```python
from build123d import *

# Parameters (mm, degrees)
SKETCH_1_R      = 2.5
EXTRUDE_1_DEPTH = 3


with BuildPart() as part:
    # 草图1 → 凸台-拉伸1 (new body)
    with BuildSketch(Plane(origin=(0, 0, 0), x_dir=(0, 0, -1), z_dir=(1, 0, 0))):
        with BuildLine():
            Line((0, -10), (175, -10))
            Line((175, -10), (200, -10))
            ThreePointArc((200, -10), (203.535533906, -8.535533906), (205, -5))
            Line((205, -5), (205, 45))
            ThreePointArc((205, 45), (204.472135955, 47.236067977), (203, 49))
            Line((203, 49), (177.666666667, 68))
            ThreePointArc((177.666666667, 68), (174.828944327, 69.486832981), (171.666666667, 70))
            Line((171.666666667, 70), (95, 70))
            ThreePointArc((95, 70), (91.207635036, 69.252997784), (87.98185108, 67.123593597))
            Line((87.98185108, 67.123593597), (32.919623175, 12.876406403))
            ThreePointArc((32.919623175, 12.876406403), (29.693839218, 10.747002216), (25.901474255, 10))
            Line((25.901474255, 10), (0, 10))
            ThreePointArc((0, 10), (-10, 0), (0, -10))
        make_face()
        Circle(SKETCH_1_R, mode=Mode.SUBTRACT)
        with Locations((95, 0)):
            Circle(SKETCH_1_R, mode=Mode.SUBTRACT)
        with Locations((95, 60)):
            Circle(SKETCH_1_R, mode=Mode.SUBTRACT)
        with Locations((200, 45)):
            Circle(SKETCH_1_R, mode=Mode.SUBTRACT)
        with Locations((200, -5)):
            Circle(SKETCH_1_R, mode=Mode.SUBTRACT)
        with Locations((185, 45)):
            Circle(SKETCH_1_R, mode=Mode.SUBTRACT)
        with Locations((185, -5)):
            Circle(SKETCH_1_R, mode=Mode.SUBTRACT)
        with BuildLine():
            Line((46.298034327, 0), (75.635083269, 0))
            ThreePointArc((75.635083269, 0), (78.696945447, 1.047152925), (80.476312452, 3.75))
            ThreePointArc((80.476312452, 3.75), (84.393398282, 10.606601718), (91.25, 14.523687548))
            ThreePointArc((91.25, 14.523687548), (93.952847075, 16.303054553), (95, 19.364916731))
            Line((95, 19.364916731), (95, 40.635083269))
            ThreePointArc((95, 40.635083269), (93.952847075, 43.696945447), (91.25, 45.476312452))
            ThreePointArc((91.25, 45.476312452), (89.208124255, 46.163303308), (87.285721083, 47.135712192))
            ThreePointArc((87.285721083, 47.135712192), (84.121274015, 47.812324342), (81.205220318, 46.409413055))
            Line((81.205220318, 46.409413055), (42.788959867, 8.561796798))
            ThreePointArc((42.788959867, 8.561796798), (41.671535435, 3.103817518), (46.298034327, 0))
        make_face(mode=Mode.SUBTRACT)
        with BuildLine():
            Line((108.2, 43.85), (121.333333333, 34))
            ThreePointArc((121.333333333, 34), (123.333333333, 30), (121.333333333, 26))
            Line((121.333333333, 26), (108.2, 16.15))
            ThreePointArc((108.2, 16.15), (106.105572809, 15.961145618), (105, 17.75))
            Line((105, 17.75), (105, 42.25))
            ThreePointArc((105, 42.25), (106.105572809, 44.038854382), (108.2, 43.85))
        make_face(mode=Mode.SUBTRACT)
        with BuildLine():
            Line((122.666666667, 50), (147.333333333, 50))
            ThreePointArc((147.333333333, 50), (149.230699929, 48.632455532), (148.533333333, 46.4))
            Line((148.533333333, 46.4), (138, 38.5))
            ThreePointArc((138, 38.5), (135, 37.5), (132, 38.5))
            Line((132, 38.5), (121.466666667, 46.4))
            ThreePointArc((121.466666667, 46.4), (120.769300071, 48.632455532), (122.666666667, 50))
        make_face(mode=Mode.SUBTRACT)
        with BuildLine():
            Line((163.201700099, 40.901275074), (163.201700099, 19.098724926))
            ThreePointArc((163.201700099, 19.098724926), (162.09612729, 17.309870544), (160.001700099, 17.498724926))
            Line((160.001700099, 17.498724926), (148.666666667, 26))
            ThreePointArc((148.666666667, 26), (146.666666667, 30), (148.666666667, 34))
            Line((148.666666667, 34), (160.001700099, 42.501275074))
            ThreePointArc((160.001700099, 42.501275074), (162.09612729, 42.690129456), (163.201700099, 40.901275074))
        make_face(mode=Mode.SUBTRACT)
        with BuildLine():
            Line((121.466666667, 13.6), (132, 21.5))
            ThreePointArc((132, 21.5), (135, 22.5), (138, 21.5))
            Line((138, 21.5), (148.533333333, 13.6))
            ThreePointArc((148.533333333, 13.6), (149.230699929, 11.367544468), (147.333333333, 10))
            Line((147.333333333, 10), (122.666666667, 10))
            ThreePointArc((122.666666667, 10), (120.769300071, 11.367544468), (121.466666667, 13.6))
        make_face(mode=Mode.SUBTRACT)
        with BuildLine():
            Line((115, 63), (165, 63))
            ThreePointArc((165, 63), (168, 60), (165, 57))
            Line((165, 57), (115, 57))
            ThreePointArc((115, 57), (112, 60), (115, 63))
        make_face(mode=Mode.SUBTRACT)
        with BuildLine():
            Line((115, 3), (165, 3))
            ThreePointArc((165, 3), (168, 0), (165, -3))
            Line((165, -3), (115, -3))
            ThreePointArc((115, -3), (112, 0), (115, 3))
        make_face(mode=Mode.SUBTRACT)
        with BuildLine():
            Line((188, 37), (197, 37))
            ThreePointArc((197, 37), (199.121320344, 36.121320344), (200, 34))
            Line((200, 34), (200, 6))
            ThreePointArc((200, 6), (199.121320344, 3.878679656), (197, 3))
            Line((197, 3), (188, 3))
            ThreePointArc((188, 3), (185.878679656, 3.878679656), (185, 6))
            Line((185, 6), (185, 34))
            ThreePointArc((185, 34), (185.878679656, 36.121320344), (188, 37))
        make_face(mode=Mode.SUBTRACT)
    extrude(amount=EXTRUDE_1_DEPTH)


solid = part.part
```
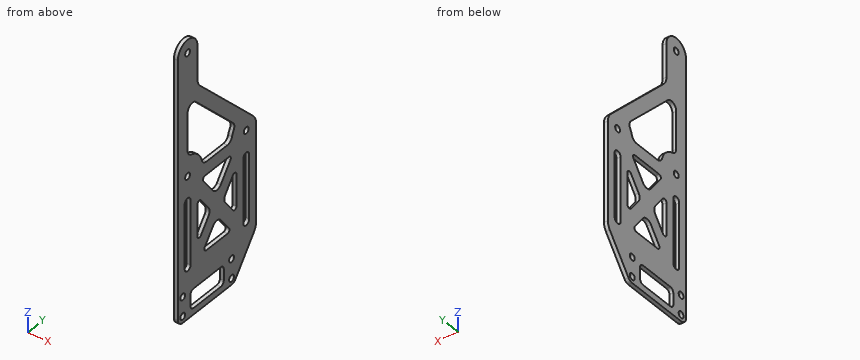
Input: part model. Units: mm. Frame: model coordinates. Round coordinates to 2 decimals unless told otherwise and drop trailing zeros. Order: outer loops, then holes, each group sorted by start corner. A loop starts at its lowest first (then second) coordinate and runs counter-clockwise, first axis right, second up. Notation, with made-up numbers: (31, 19) - (65, 19) arc R31 ccw to (65, 49) - close; hole circle Ø11 at (-11, 86.25). An arc over 180 degrees is marked (long way). Answer in a Markdown table with one row per item.
Item 1: Pin query (flat end, axial travel): pin 1 (1.5 mm diameter, centred on x = 2.5, y = 44.5, fed in from +Z); pin 2 (1.5 mm diameter, centred on x = 2.5, y = 52.5, fed in from -Z); pin 3 (1.5 mm diameter, centred on x = 2, z = -7, fed in from +Y); pin 4 (3 mm diameter, centred on y = 0, z = -95, fed in from +X). Return the tip coordinate at first contact, or that it passes through.
Model answer:
| item | result |
|---|---|
| pin 1 | stops at z = -64.26 |
| pin 2 | stops at z = -199.33 |
| pin 3 | stops at y = 10 |
| pin 4 | passes through |
Item 2: Line query: line 1 (Z direction, x = 0.6, y = 4); line 2 (Z direction, x = 2, y = -2); line 3 (Z direction, x = 0.7, y = 44). Output: solid intervals per line, ascending.
Model answer:
| item | result |
|---|---|
| line 1 | z = -205 to -199.24, -185.76 to -80.54, -41.4 to 9.17 |
| line 2 | z = -205 to -167.24, -112.76 to -96.5, -93.5 to -1.5, 1.5 to 9.8 |
| line 3 | z = -205 to -202.29, -197.71 to -187.29, -182.71 to -145.33, -124.67 to -107.97, -106.03 to -93.7, -78.76 to -64.51 |
Item 3: Section query A-A (z = -144). Return the cut outline in (x, y).
Model answer:
| item | result |
|---|---|
| outline | (0, -10) - (3, -10) - (3, -3) - (0, -3) - close; (0, 3) - (3, 3) - (3, 10) - (0, 10) - close; (0, 17) - (3, 17) - (3, 43) - (0, 43) - close; (0, 50) - (3, 50) - (3, 57) - (0, 57) - close; (0, 63) - (3, 63) - (3, 70) - (0, 70) - close |
Item 4: Section query B-B (x = 0.9). Give the number of separate pieces and of enclosed holes in the cut face, then the cut area to 3 significant figures.
Model answer:
| item | result |
|---|---|
| separate pieces | 1 |
| enclosed holes | 15 |
| area | 8,690 mm² |
